```python
from build123d import *

# Parameters (mm, degrees)
BOSS_EXTRUDE1_DEPTH = 1.5
BOSS_EXTRUDE2_START = 4
SKETCH2_R           = 1.75
SKETCH2_W           = 6
SKETCH2_H           = 10
BOSS_EXTRUDE2_DEPTH = 4
FILLET1_R           = 1.75
SKETCH4_R           = 1.5
BOSS_EXTRUDE4_DEPTH = 3.5
FILLET2_R           = 1
SKETCH5_R           = 2
CUT_EXTRUDE1_DEPTH  = 3.75
BOSS_EXTRUDE5_DEPTH = 2
BOSS_EXTRUDE6_DEPTH = 6


with BuildPart() as part:
    # Sketch1 → Boss-Extrude1 (new body)
    with BuildSketch(Plane(origin=(0, 0, 0), x_dir=(1, 0, 0), z_dir=(0, 1, 0))):
        with BuildLine():
            Line((5, 5), (11, 5))
            Line((11, 5), (11, -5))
            Line((11, -5), (5, -5))
            Line((5, -5), (-0.892691591, -1.505191591))
            ThreePointArc((-0.892691591, -1.505191591), (-1.75, 0), (-0.892691591, 1.505191591))
            Line((-0.892691591, 1.505191591), (5, 5))
        make_face()
    extrude(amount=-BOSS_EXTRUDE1_DEPTH)

    # Sketch2 → Boss-Extrude2 (add)
    with BuildSketch(Plane(origin=(0, 0, 0), x_dir=(1, 0, 0), z_dir=(0, 1, 0)).offset(BOSS_EXTRUDE2_START)):
        with Locations(Location((0, 0, 0), (0, 0, 270))):
            Circle(SKETCH2_R)
        with Locations((8, 0)):
            Rectangle(SKETCH2_W, SKETCH2_H)
    extrude(amount=-BOSS_EXTRUDE2_DEPTH)

    # Fillet1
    fillet1_edges = [part.edges().sort_by_distance(p)[0] for p in [
        (0, 4, -1.75),
    ]]
    fillet(fillet1_edges, radius=FILLET1_R)

    # Sketch4 → Boss-Extrude4 (add)
    with BuildSketch(Plane(origin=(0, 4, 0), x_dir=(1, 0, 0), z_dir=(0, 1, 0))):
        with Locations(Location((8, 2.5, 0), (0, 0, 270))):
            Circle(SKETCH4_R)
    extrude(amount=BOSS_EXTRUDE4_DEPTH)

    # Fillet2
    fillet2_edges = [part.edges().sort_by_distance(p)[0] for p in [
        (8, 7.5, -4),
    ]]
    fillet(fillet2_edges, radius=FILLET2_R)

    # Sketch5 → Cut-Extrude1 (cut)
    with BuildSketch(Plane(origin=(0, 4, 0), x_dir=(1, 0, 0), z_dir=(0, 1, 0))):
        with Locations(Location((8, -2.5, 0), (0, 0, 270))):
            Circle(SKETCH5_R)
    extrude(amount=-CUT_EXTRUDE1_DEPTH, mode=Mode.SUBTRACT)

    # Sketch6 → Boss-Extrude5 (add)
    with BuildSketch(Plane(origin=(11, 0, 0), x_dir=(0, 0, -1), z_dir=(1, 0, 0))):
        with BuildLine():
            Line((-2, 4), (2, 4))
            ThreePointArc((2, 4), (0, 2), (-2, 4))
        make_face()
    extrude(amount=BOSS_EXTRUDE5_DEPTH)

    # Sketch9 → Boss-Extrude6 (add)
    with BuildSketch(Plane(origin=(11, 0, 0), x_dir=(0, 0, -1), z_dir=(1, 0, 0))):
        Polygon((-5, 4), (-8.7, 4), (-5, 0.3), align=None)
        Polygon((5, 0.3), (5, 4), (8.7, 4), align=None)
    extrude(amount=-BOSS_EXTRUDE6_DEPTH)


solid = part.part
```
The listing builds one solid part. Answer for the finished solid, in the listing's coordinates (mm). A direction names the side the tool comes from. Coordinates: 2 decimals unless noted, no trailing zeros. Loops run counter-clockwise (first coordinate to the right, second up) from the corner with the lowest first, then second, coordinate; pieces in that order, holes last. Notation, with made-up numbers: (-19, -17) - (17, -17) arc R27 ccw to (17, 7) - close; hole circle Ø7 at (64.5, -21.75). An arc over 180 degrees is marked (long way). Use a Markdown table: item, result. Add a question column.
1) Find the intervals of material crossed by line 1 (X direction, y = 2.3, z = 2.5); line 2 (Z direction, x = 6.5, y = 3.75); line 3 (Z direction, x = 7.5, y = -0.25), in increasing order.
2) The mould has two halves that part along X. Classify faces 6 (the flat face through (11, 1, 0)), 7 (the cylindrical face through (9.983, 2.151, 2.24)), 8 (the flat face through (8, -1, 5)): released by +X, released by -X, zero draft, split by the parting line, or undercut.
3) The part is cut by section D-D, the plane z = -4.25. Give the vertices of the cut face in (x, y), and give its area (3 significant figures).
4) The part is cut by section C-C, the plane x = 0. Give the vertices of the cut face in (y, z), and give its area (3 significant figures).
5) The part is cut by section A-A, the plane z = 3.5. Give the vertices of the cut face in (x, y), and give its area (3 significant figures).
6) The part is cut by section B-B, the plane y = -0.25. Give the vertices of the cut face in (x, z).
7) For faces 1 (the cylindrical face through (12, 2, 0)), 2 (the flat face through (8, -1, -5)), 3 (the flat face through (5, 2, 0)), 4 (the flat face through (8, 0.25, 2)), 5 (the flat face through (13, 3, 0)), determine the directions among +Z, -Z, +X, -X, +Y, -Y from which every point of the face is accessible in a straight line to the end or side of a thin tool.
8) Given pin 1 (4 mm diameter, centred on x = 8.5, z = -2, fed in from +Y); pin 2 (3 mm diameter, centred on y = 2.5, z = -6, fed in from +X); pin 3 (1.4 mm diameter, centred on x = 9, y = -0.5, fed in from +Z); pin 4 (1.8 mm diameter, centred on x = 1, z = 1, fed in from +Y), each flat-ended and moving along its own axis, determine where each tip first touches the part or whether it passes through.
Here are the results:
| question | item | result |
|---|---|---|
| 1 | line 1 | x = 5 to 6, 10 to 11 |
| 1 | line 2 | z = -8.45 to 1.18, 3.82 to 8.45 |
| 1 | line 3 | z = -5 to 5 |
| 2 | face 6 | released by +X |
| 2 | face 7 | undercut |
| 2 | face 8 | zero draft |
| 3 | outline | (3.74, -1.5) - (11, -1.5) - (11, 4) - (5, 4) - (5, 0) - (3.74, 0) - close |
| 3 | area | 34.9 mm^2 |
| 4 | outline | (-1.5, -2.03) - (0, -2.03) - (0, -1.75) - (2.25, -1.75) arc R1.75 ccw to (2.25, 1.75) - (0, 1.75) - (0, 2.03) - (-1.5, 2.03) - close |
| 4 | area | 18.8 mm^2 |
| 5 | outline | (2.47, -1.5) - (11, -1.5) - (11, 4) - (9.73, 4) - (9.73, 0.25) - (6.27, 0.25) - (6.27, 4) - (5, 4) - (5, 0) - (2.47, 0) - close |
| 5 | area | 23.8 mm^2 |
| 6 | outline | (-0.89, -1.51) - (5, -5) - (11, -5) - (11, 5) - (5, 5) - (-0.89, 1.51) arc R1.75 ccw to start |
| 7 | face 1 | +X, -Y |
| 7 | face 2 | -Z, +X, -X, -Y |
| 7 | face 3 | +Z, -Z, +Y |
| 7 | face 4 | +Y |
| 7 | face 5 | +Z, -Z, +X, +Y, -Y |
| 8 | pin 1 | stops at y = 7.5 |
| 8 | pin 2 | stops at x = 11 |
| 8 | pin 3 | stops at z = 5 |
| 8 | pin 4 | stops at y = 3.92 |
